Check sheet for the modelled part. Datum: model origin and axes. Units: mm. A direction names the side the tool comes from. Give positions to 0.01 mm unless a question says otherwise; leave off trailing zeros. Order: outer loops, then holes, each group sorted by start corner. A loop starts at its lowest first (then second) coordinate and runs counter-clockwise, first axis right, second up.
Item 1: Material ranges on line 1 along X through (y, z) = (-24, 2.45); line 2 along Y through (x, z) = (0, 0.75); line 3 along Y through (x, z) = (-11.5, 2.25), recorded low to high.
Item 2: Sectioned sample at D-D on y = -19. Record the boundary of the cut face in (x, z).
Item 3: Sectioned sample at B-B on x = -11.5. Record the boundary of the cut face in (y, z), and give its area (3 significant figures).
Item 4: Gauge pin test, flat ends, axial feed: P1, Ø0.9, axis at y = -9, z = 2, coming from the -X side; P2, Ø2.5, axis at x = 0, y = -8, coming from the -Z side; P3, Ø1.5, axis at y = 17.5, z = 1, coming from the +X side. Record the tip position at first contact, or that the pin passes through.
Item 5: Sectioned sample at C-C on y = 24. Record the boundary of the cut face in (x, z), and give its area (3 significant figures).
Item 6: Sectioned sample at A-A on y = 8. Record the boundary of the cut face in (x, z).
Item 7: Access from +Z, -Z, +X, -X, +Y, -Y to the whole of each face (thin tool, end or side, straight path). Record for faces 1 (the flat face through (16, 24, 1)), 2 (the flat face through (-1.5, 0, 1)).
from build123d import *

# Parameters (mm, degrees)
SKETCH_1_W                = 32
SKETCH_1_H                = 64
EXTRUDE_1_DEPTH           = 3
SKETCH_2_W                = 2.5
SKETCH_2_H                = 4
CUT_EXTRUDE_1_DEPTH       = 36.902646142
MIRROR_2_COPY_1_SKETCH_W  = 2.5
MIRROR_2_COPY_1_SKETCH_H  = 4
MIRROR_2_COPY_1_DEPTH     = 36.902646142
SKETCH_4_W                = 3
SKETCH_4_H                = 8
CUT_EXTRUDE_3_DEPTH       = 10
SKETCH_6_W                = 3
SKETCH_6_H                = 4
CUT_EXTRUDE_5_DEPTH       = 36.902646142
MIRROR_9_COPY_1_SKETCH_W  = 3
MIRROR_9_COPY_1_SKETCH_H  = 4
MIRROR_9_COPY_1_DEPTH     = 36.902646142
SKETCH_8_R                = 1.5
CUT_EXTRUDE_6_DEPTH       = 36.902646142
MIRROR_11_COPY_1_SKETCH_R = 1.5
MIRROR_11_COPY_1_DEPTH    = 36.902646142
SKETCH_10_R               = 1.5
CUT_EXTRUDE_8_DEPTH       = 36.902646142
MIRROR_15_COPY_1_SKETCH_R = 1.5
MIRROR_15_COPY_1_DEPTH    = 36.902646142
SKETCH_11_R               = 1.5
CUT_EXTRUDE_9_DEPTH       = 36.902646142
MIRROR_17_COPY_1_SKETCH_R = 1.5
MIRROR_17_COPY_1_DEPTH    = 36.902646142
SKETCH_12_W               = 3
SKETCH_12_H               = 8
CUT_EXTRUDE_10_DEPTH      = 36.902646142
MIRROR_19_COPY_1_SKETCH_W = 3
MIRROR_19_COPY_1_SKETCH_H = 8
MIRROR_19_COPY_1_DEPTH    = 36.902646142
SKETCH_13_R               = 1.5
CUT_EXTRUDE_11_DEPTH      = 36.902646142
MIRROR_21_COPY_1_SKETCH_R = 1.5
MIRROR_21_COPY_1_DEPTH    = 36.902646142
SKETCH_14_W               = 5
SKETCH_14_H               = 8
CUT_EXTRUDE_12_DEPTH      = 36.902646142
SKETCH_15_R               = 1.5
CUT_EXTRUDE_13_DEPTH      = 36.902646142
EXTRUDE_START             = -3
SKETCH_16_R               = 1.5
EXTRUDE_2_DEPTH           = 3
SKETCH_17_R               = 1.5
EXTRUDE_3_DEPTH           = 3
SKETCH_18_W               = 3.452729718
SKETCH_18_H               = 30.432996322
SKETCH_18_W_2             = 3.815279569
CUT_EXTRUDE_14_DEPTH      = 36.902646142


with BuildPart() as part:
    # 草图1 → 凸台-拉伸1 (new body)
    with BuildSketch(Plane.XY):
        Rectangle(SKETCH_1_W, SKETCH_1_H)
    extrude(amount=EXTRUDE_1_DEPTH)

    # 草图2 → 切除-拉伸1 (cut, through all)
    with BuildSketch(Plane.XY.offset(3)):
        Polygon((4, 16), (4, 12), (6.5, 12), (6.5, 20), (1.5, 20), (1.5, 16), align=None)
        with Locations((2.75, 14)):
            Rectangle(SKETCH_2_W, SKETCH_2_H)
    cut_extrude_1 = extrude(amount=-CUT_EXTRUDE_1_DEPTH, mode=Mode.SUBTRACT)

    # 镜向1: 切除-拉伸1 across plane
    add(cut_extrude_1.mirror(Plane(origin=(0, 0, 0), x_dir=(0, 0, 1), z_dir=(1, 0, 0))), mode=Mode.SUBTRACT)

    # 镜向2: 切除-拉伸1 across plane
    add(cut_extrude_1.mirror(Plane.ZX), mode=Mode.SUBTRACT)

    # 镜向2 copy 1 sketch → 镜向2 copy 1 (cut, through all)
    with BuildSketch(Plane(origin=(0, 0, 3), x_dir=(-1, 0, 0), z_dir=(0, 0, 1))):
        Polygon((4, 16), (4, 12), (6.5, 12), (6.5, 20), (1.5, 20), (1.5, 16), align=None)
        with Locations((2.75, 14)):
            Rectangle(MIRROR_2_COPY_1_SKETCH_W, MIRROR_2_COPY_1_SKETCH_H)
    extrude(amount=-MIRROR_2_COPY_1_DEPTH, mode=Mode.SUBTRACT)

    # 草图4 → 切除-拉伸3 (cut)
    with BuildSketch(Plane.XY.offset(3)):
        with Locations((14.5, 0)):
            Rectangle(SKETCH_4_W, SKETCH_4_H)
    cut_extrude_3 = extrude(amount=-CUT_EXTRUDE_3_DEPTH, mode=Mode.SUBTRACT)

    # 镜向5: 切除-拉伸3 across plane
    add(cut_extrude_3.mirror(Plane(origin=(0, 0, 0), x_dir=(0, 0, 1), z_dir=(1, 0, 0))), mode=Mode.SUBTRACT)

    # 草图6 → 切除-拉伸5 (cut, through all)
    with BuildSketch(Plane.XY.offset(3)):
        with Locations((14.5, 30)):
            Rectangle(SKETCH_6_W, SKETCH_6_H)
    cut_extrude_5 = extrude(amount=-CUT_EXTRUDE_5_DEPTH, mode=Mode.SUBTRACT)

    # 镜向8: 切除-拉伸5 across plane
    add(cut_extrude_5.mirror(Plane.ZX), mode=Mode.SUBTRACT)

    # 镜向9: 切除-拉伸5 across plane
    add(cut_extrude_5.mirror(Plane(origin=(0, 0, 0), x_dir=(0, 0, 1), z_dir=(1, 0, 0))), mode=Mode.SUBTRACT)

    # 镜向9 copy 1 sketch → 镜向9 copy 1 (cut, through all)
    with BuildSketch(Plane(origin=(0, 0, 3), x_dir=(-1, 0, 0), z_dir=(0, 0, 1))):
        with Locations((14.5, 30)):
            Rectangle(MIRROR_9_COPY_1_SKETCH_W, MIRROR_9_COPY_1_SKETCH_H)
    extrude(amount=-MIRROR_9_COPY_1_DEPTH, mode=Mode.SUBTRACT)

    # 草图8 → 切除-拉伸6 (cut, through all)
    with BuildSketch(Plane.XY.offset(3)):
        with Locations((14, 29)):
            Circle(SKETCH_8_R)
    cut_extrude_6 = extrude(amount=-CUT_EXTRUDE_6_DEPTH, mode=Mode.SUBTRACT)

    # 镜向10: 切除-拉伸6 across plane
    add(cut_extrude_6.mirror(Plane(origin=(0, 0, 0), x_dir=(0, 0, 1), z_dir=(1, 0, 0))), mode=Mode.SUBTRACT)

    # 镜向11: 切除-拉伸6 across plane
    add(cut_extrude_6.mirror(Plane.ZX), mode=Mode.SUBTRACT)

    # 镜向11 copy 1 sketch → 镜向11 copy 1 (cut, through all)
    with BuildSketch(Plane(origin=(0, 0, 3), x_dir=(-1, 0, 0), z_dir=(0, 0, 1))):
        with Locations((14, 29)):
            Circle(MIRROR_11_COPY_1_SKETCH_R)
    extrude(amount=-MIRROR_11_COPY_1_DEPTH, mode=Mode.SUBTRACT)

    # 草图10 → 切除-拉伸8 (cut, through all)
    with BuildSketch(Plane.XY.offset(3)):
        with Locations((-14, 3)):
            Circle(SKETCH_10_R)
    cut_extrude_8 = extrude(amount=-CUT_EXTRUDE_8_DEPTH, mode=Mode.SUBTRACT)

    # 镜向14: 切除-拉伸8 across plane
    add(cut_extrude_8.mirror(Plane.ZX), mode=Mode.SUBTRACT)

    # 镜向15: 切除-拉伸8 across plane
    add(cut_extrude_8.mirror(Plane(origin=(0, 0, 0), x_dir=(0, 0, 1), z_dir=(1, 0, 0))), mode=Mode.SUBTRACT)

    # 镜向15 copy 1 sketch → 镜向15 copy 1 (cut, through all)
    with BuildSketch(Plane(origin=(0, 0, 3), x_dir=(-1, 0, 0), z_dir=(0, 0, 1))):
        with Locations((-14, 3)):
            Circle(MIRROR_15_COPY_1_SKETCH_R)
    extrude(amount=-MIRROR_15_COPY_1_DEPTH, mode=Mode.SUBTRACT)

    # 草图11 → 切除-拉伸9 (cut, through all)
    with BuildSketch(Plane.XY.offset(3)):
        with Locations((-11.5, 8)):
            Circle(SKETCH_11_R)
        with Locations((-11.5, 24)):
            Circle(SKETCH_11_R)
    cut_extrude_9 = extrude(amount=-CUT_EXTRUDE_9_DEPTH, mode=Mode.SUBTRACT)

    # 镜向16: 切除-拉伸9 across plane
    add(cut_extrude_9.mirror(Plane(origin=(0, 0, 0), x_dir=(0, 0, 1), z_dir=(1, 0, 0))), mode=Mode.SUBTRACT)

    # 镜向17: 切除-拉伸9 across plane
    add(cut_extrude_9.mirror(Plane.ZX), mode=Mode.SUBTRACT)

    # 镜向17 copy 1 sketch → 镜向17 copy 1 (cut, through all)
    with BuildSketch(Plane(origin=(0, 0, 3), x_dir=(-1, 0, 0), z_dir=(0, 0, 1))):
        with Locations((-11.5, 8)):
            Circle(MIRROR_17_COPY_1_SKETCH_R)
        with Locations((-11.5, 24)):
            Circle(MIRROR_17_COPY_1_SKETCH_R)
    extrude(amount=-MIRROR_17_COPY_1_DEPTH, mode=Mode.SUBTRACT)

    # 草图12 → 切除-拉伸10 (cut, through all)
    with BuildSketch(Plane(origin=(0, 0, 0), x_dir=(-1, 0, 0), z_dir=(0, 0, -1))):
        with Locations((-14.5, 16)):
            Rectangle(SKETCH_12_W, SKETCH_12_H)
    cut_extrude_10 = extrude(amount=-CUT_EXTRUDE_10_DEPTH, mode=Mode.SUBTRACT)

    # 镜向18: 切除-拉伸10 across plane
    add(cut_extrude_10.mirror(Plane(origin=(0, 0, 0), x_dir=(0, 0, 1), z_dir=(1, 0, 0))), mode=Mode.SUBTRACT)

    # 镜向19: 切除-拉伸10 across plane
    add(cut_extrude_10.mirror(Plane.ZX), mode=Mode.SUBTRACT)

    # 镜向19 copy 1 sketch → 镜向19 copy 1 (cut, through all)
    with BuildSketch(Plane(origin=(0, 0, 0), x_dir=(1, 0, 0), z_dir=(0, 0, -1))):
        with Locations((-14.5, 16)):
            Rectangle(MIRROR_19_COPY_1_SKETCH_W, MIRROR_19_COPY_1_SKETCH_H)
    extrude(amount=-MIRROR_19_COPY_1_DEPTH, mode=Mode.SUBTRACT)

    # 草图13 → 切除-拉伸11 (cut, through all)
    with BuildSketch(Plane(origin=(0, 0, 0), x_dir=(-1, 0, 0), z_dir=(0, 0, -1))):
        with Locations((-14, 19)):
            Circle(SKETCH_13_R)
        with Locations((-14, 13)):
            Circle(SKETCH_13_R)
    cut_extrude_11 = extrude(amount=-CUT_EXTRUDE_11_DEPTH, mode=Mode.SUBTRACT)

    # 镜向20: 切除-拉伸11 across plane
    add(cut_extrude_11.mirror(Plane(origin=(0, 0, 0), x_dir=(0, 0, 1), z_dir=(1, 0, 0))), mode=Mode.SUBTRACT)

    # 镜向21: 切除-拉伸11 across plane
    add(cut_extrude_11.mirror(Plane.ZX), mode=Mode.SUBTRACT)

    # 镜向21 copy 1 sketch → 镜向21 copy 1 (cut, through all)
    with BuildSketch(Plane(origin=(0, 0, 0), x_dir=(1, 0, 0), z_dir=(0, 0, -1))):
        with Locations((-14, 19)):
            Circle(MIRROR_21_COPY_1_SKETCH_R)
        with Locations((-14, 13)):
            Circle(MIRROR_21_COPY_1_SKETCH_R)
    extrude(amount=-MIRROR_21_COPY_1_DEPTH, mode=Mode.SUBTRACT)

    # 草图14 → 切除-拉伸12 (cut, through all)
    with BuildSketch(Plane(origin=(0, 0, 0), x_dir=(-1, 0, 0), z_dir=(0, 0, -1))):
        with Locations((4, 0)):
            Rectangle(SKETCH_14_W, SKETCH_14_H)
    cut_extrude_12 = extrude(amount=-CUT_EXTRUDE_12_DEPTH, mode=Mode.SUBTRACT)

    # 镜向22: 切除-拉伸12 across plane
    add(cut_extrude_12.mirror(Plane(origin=(0, 0, 0), x_dir=(0, 0, 1), z_dir=(1, 0, 0))), mode=Mode.SUBTRACT)

    # 草图15 → 切除-拉伸13 (cut, through all)
    with BuildSketch(Plane(origin=(0, 0, 0), x_dir=(-1, 0, 0), z_dir=(0, 0, -1))):
        with Locations((0, 8)):
            Circle(SKETCH_15_R)
        with Locations((0, 24)):
            Circle(SKETCH_15_R)
    cut_extrude_13 = extrude(amount=-CUT_EXTRUDE_13_DEPTH, mode=Mode.SUBTRACT)

    # 镜向23: 切除-拉伸13 across plane
    add(cut_extrude_13.mirror(Plane.ZX), mode=Mode.SUBTRACT)

    # 草图16 → 凸台-拉伸2 (add)
    with BuildSketch(Plane(origin=(0, 0, 0), x_dir=(-1, 0, 0), z_dir=(0, 0, -1)).offset(EXTRUDE_START)):
        with Locations((-11.5, 8)):
            Circle(SKETCH_16_R)
        with Locations((11.5, 8)):
            Circle(SKETCH_16_R)
        with Locations((11.5, -8)):
            Circle(SKETCH_16_R)
        with Locations((-11.5, -8)):
            Circle(SKETCH_16_R)
    extrude(amount=EXTRUDE_2_DEPTH)

    # 草图17 → 凸台-拉伸3 (add)
    with BuildSketch(Plane(origin=(0, 0, 0), x_dir=(-1, 0, 0), z_dir=(0, 0, -1))):
        with Locations((14, 13)):
            Circle(SKETCH_17_R)
        with Locations((-14, 13)):
            Circle(SKETCH_17_R)
        with Locations((-14, 3)):
            Circle(SKETCH_17_R)
        with Locations((14, 3)):
            Circle(SKETCH_17_R)
        with Locations((14, -3)):
            Circle(SKETCH_17_R)
        with Locations((-14, -3)):
            Circle(SKETCH_17_R)
        with Locations((-14, -13)):
            Circle(SKETCH_17_R)
        with Locations((14, -13)):
            Circle(SKETCH_17_R)
    extrude(amount=-EXTRUDE_3_DEPTH)

    # 草图18 → 切除-拉伸14 (cut, through all)
    with BuildSketch(Plane(origin=(0, 0, 0), x_dir=(-1, 0, 0), z_dir=(0, 0, -1))):
        with Locations((14.726364859, 0.092049044)):
            Rectangle(SKETCH_18_W, SKETCH_18_H)
        with Locations((-14.907639785, 0.092049044)):
            Rectangle(SKETCH_18_W_2, SKETCH_18_H)
    extrude(amount=-CUT_EXTRUDE_14_DEPTH, mode=Mode.SUBTRACT)


solid = part.part
Report:
1. line 1: x = -16 to -13, -10 to -1.5, 1.5 to 10, 13 to 16
1. line 2: y = -32 to -25.5, -22.5 to -9.5, -6.5 to 6.5, 9.5 to 22.5, 25.5 to 32
1. line 3: y = -32 to -25.5, -22.5 to 22.5, 25.5 to 32
2. outline: (-12.5, 0) - (-6.5, 0) - (-6.5, 3) - (-12.5, 3) - close; (-1.5, 0) - (1.5, 0) - (1.5, 3) - (-1.5, 3) - close; (6.5, 0) - (12.5, 0) - (12.5, 3) - (6.5, 3) - close
3. outline: (-32, 0) - (-25.5, 0) - (-25.5, 3) - (-32, 3) - close; (-22.5, 0) - (22.5, 0) - (22.5, 3) - (-22.5, 3) - close; (25.5, 0) - (32, 0) - (32, 3) - (25.5, 3) - close
3. area: 174 mm2
4. P1: stops at x = -13
4. P2: passes through
4. P3: stops at x = 13
5. outline: (-16, 0) - (-13, 0) - (-13, 3) - (-16, 3) - close; (-10, 0) - (-1.5, 0) - (-1.5, 3) - (-10, 3) - close; (1.5, 0) - (10, 0) - (10, 3) - (1.5, 3) - close; (13, 0) - (16, 0) - (16, 3) - (13, 3) - close
5. area: 69.0 mm2
6. outline: (-13, 0) - (-1.5, 0) - (-1.5, 3) - (-13, 3) - close; (1.5, 0) - (13, 0) - (13, 3) - (1.5, 3) - close
7. face 1: +Z, -Z, +X, +Y, -Y
7. face 2: +Z, -Z
